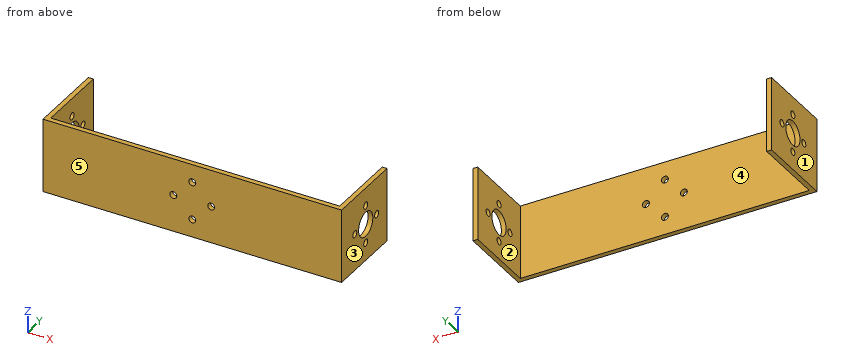
Autodesk Inventor part; units mm, degrees
ref_plane "YZ Plane" through (0, 0, 0) normal (1, 0, 0) x (0, 1, 0)
ref_plane "XZ Plane" through (0, 0, 0) normal (0, 1, 0) x (-1, 0, 0)
ref_plane "XY Plane" through (0, 0, 0) normal (0, 0, 1) x (1, 0, 0)
sketch "Sketch1" plane through (0, 0, 0) normal (0, 1, 0) x (-1, 0, 0)
  line L0 (0, 0) -> (154.0002, 0)
  line L1 (154.0002, 0) -> (154.0002, -38.1)
  line L2 (154.0002, -38.1) -> (0, -38.1)
  line L3 (0, -38.1) -> (0, 0)
  dimension "d0" = 154.0002
  dimension "d1" = 38.1
extrude "Extrusion1" add sketch "Sketch1" along normal blind 2.54
sketch "Sketch3" plane through (0, 0, 0) normal (1, 0, 0) x (0, 0, -1)
  circle A0 centre (19.05, 31.369) radius 1.7907
  circle A1 centre (28.829, 21.59) radius 1.7907
  circle A2 centre (19.05, 11.811) radius 1.7907
  circle A3 centre (9.271, 21.59) radius 1.7907
  circle A4 centre (19.05, 21.59) radius 6.35
  point P0 (0, 0)
  dimension "d12" = 12.7
sketch "Sketch4" plane through (0, 2.54, 0) normal (0, 1, 0) x (1, 0, 0)
  line L0 (0, 38.1) -> (-154.0002, 38.1)
  line L1 (0, 0) -> (-2.451, 0)
  line L2 (-2.451, 0) -> (-2.451, 38.1)
  line L3 (-2.451, 38.1) -> (0, 38.1)
  line L4 (0, 38.1) -> (0, 0)
  line L5 (-154.0002, 38.1) -> (-154.0002, 0)
  line L6 (-154.0002, 0) -> (-151.4602, 0)
  line L7 (-151.4602, 0) -> (-151.4602, 38.1)
  line L8 (-151.4602, 38.1) -> (-154.0002, 38.1)
  line L9 (-154.0002, 38.1) -> (-154.0002, 0)
  point P0 (0, 38.1)
  point P1 (-151.4602, 38.1)
  dimension "d17" = 2.54
extrude "Extrusion3" add sketch "Sketch4" along normal blind 38.1
extrude "Extrusion4" cut sketch "Sketch3" against normal blind 203.2
sketch "Sketch5" plane through (0, 2.54, 0) normal (0, 1, 0) x (1, 0, 0)
  line L0 (0, 20.8407) -> (0, 17.2593)
  line L1 (-154.0002, 38.1) -> (-154.0002, 0)
  line L2 (-77.0001, 38.1) -> (-77.0001, 0)
  line L3 (-77.0001, 19.05) -> (-154.0002, 19.05)
  circle A0 centre (-77.0001, 19.05) radius 9.779
  circle A1 centre (-86.7791, 19.05) radius 1.7907
  circle A2 centre (-77.0001, 9.271) radius 1.7907
  circle A3 centre (-77.0001, 28.829) radius 1.7907
  circle A4 centre (-67.2211, 19.05) radius 1.7907
  point P0 (0, 0)
  dimension "d18" = 19.558
  dimension "d19" = 3.5814
  dimension "d20" = 3.5814
  dimension "d21" = 3.5814
  dimension "d22" = 3.5814
extrude "Extrusion5" cut sketch "Sketch5" against normal blind 203.2 contours A3 A0 L2 | L2 A0 A3 | A0 A3 L2 | L2 A3 A0 | A1 L3 A0 | A0 L3 A1 | A4 A0 | A0 A4 | A0 A1 L3 | L3 A1 A0 | A2 A0 L2 | L2 A0 A2 | A0 A2 L2 | L2 A2 A0
properties part number "Rotate Brace"
CAD build for the part. Positions are in the model's coordinates, mm. Face numbers are marked on the shaded views. A direction names the side the tool comes from. Round coordinates to 2 decimals unless told otherwise and drop trailing zeros. Write each loop counter-clockwise with the first axis right and the second up, starting at its lowest first coordinate (ties: lowest second). Pieces come first, ordered by that corner, then holes.
(1) Drop flat-ended pins along their axis: P1, Ø1.5, axis at x = -106.5, z = -33, coming from the -Y side; P2, Ø19, axis at x = -88, z = -18, coming from the +Y side. Give the stop position or say it passes through.
(2) 3-axis set-ups, long thin cutter, end or side, ignore diameter. For the marked faces 1 and 2: which of +Z, -Z, +X, -X, +Y, -Y reach the whole face in a straight line?
(3) Slice it at A-A, the plane y = 8. Write the cut outline in (x, z), and give its area (3 significant figures).
(4) Probe line 1 along Y through (x, z) = (-1.35, -19.05); line 2 along X through (y, z) = (11.5, -23.5); line 3 along Y through (x, z) = (-26, -16). List the from-to ranges inside material, lowest first.
(5) Slice it at D-D, the plane z = -5.5. Write the cut outline in (x, y).
(6) Slice it at B-B, the plane y = 21.59. Count the separate pieces of the cut face and the enclosed holes in it, and give its area (3 significant figures).
(7) Mould opens along X. For the marked faces 3, 4 and 5 say: pulls with the +X half, pulls with the -X half, needs draft (parallel to the pull), parting line crosses it, or undercut.
From the geometry:
1. P1: stops at y = 0
1. P2: stops at y = 2.54
2. face 1: +Z, -Z, -X, +Y, -Y
2. face 2: +Z, -Z, +Y
3. outline: (-154, -38.1) - (-151.46, -38.1) - (-151.46, 0) - (-154, 0) - close; (-2.45, -38.1) - (0, -38.1) - (0, 0) - (-2.45, 0) - close
3. area: 190 mm2
4. line 1: y = 0 to 10.02, 13.6 to 15.24, 27.94 to 29.58, 33.16 to 40.64
4. line 2: x = -154 to -151.46, -2.45 to 0
4. line 3: y = 0 to 2.54
5. outline: (-154, 0) - (0, 0) - (0, 40.64) - (-2.45, 40.64) - (-2.45, 2.54) - (-151.46, 2.54) - (-151.46, 40.64) - (-154, 40.64) - close
6. separate pieces: 8
6. enclosed holes: 0
6. area: 91.0 mm2
7. face 3: pulls with the +X half
7. face 4: undercut
7. face 5: needs draft
